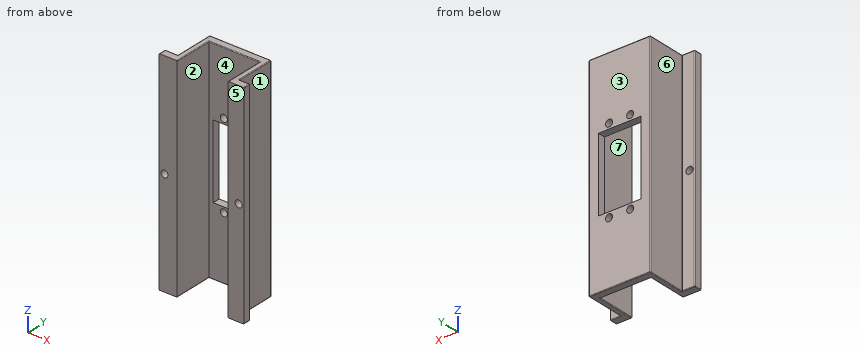
Autodesk Inventor part; units mm, degrees
ref_plane "YZ Plane" through (0, 0, 0) normal (1, 0, 0) x (0, 1, 0)
ref_plane "XZ Plane" through (0, 0, 0) normal (0, 1, 0) x (-1, 0, 0)
ref_plane "XY Plane" through (0, 0, 0) normal (0, 0, 1) x (1, 0, 0)
sketch "Sketch1" plane through (0, 0, 0) normal (0, 1, 0) x (-1, 0, 0)
  line L0 (-40, 0) -> (-40, -100)
  line L1 (0, -100) -> (0, 0)
  line L2 (-35, 0) -> (-35, -100)
  line L3 (-6, -100) -> (-6, 0)
  circle A0 centre (-2.5, -50) radius 1.65
  circle A1 centre (-37.5, -50) radius 1.65
  line L4 (0, 0) -> (-8.5, 0)
  line L5 (-32.5, 0) -> (-40, 0)
  line L6 (-40, -100) -> (-32.5, -100)
  line L7 (-8.5, -100) -> (0, -100)
  line L8 (-8.5, 0) -> (-8.5, -100)
  line L9 (-32.5, -100) -> (-32.5, 0)
  dimension "d4" = 3.3
  dimension "d5" = 3.3
  dimension "d8" = 2.5
  dimension "d9" = 2.5
extrude "Extrusion1" add sketch "Sketch1" along normal blind 3.5
sketch "Sketch2" plane through (0, 3.5, 0) normal (0, 1, 0) x (1, 0, 0)
  line L0 (8.5, 100) -> (0, 100)
  line L1 (8.5, 100) -> (6, 100)
  line L2 (6, 100) -> (6, 0)
  line L3 (6, 0) -> (8.5, 0)
  line L4 (8.5, 0) -> (8.5, 100)
  line L5 (32.5, 100) -> (32.5, 0)
  line L6 (32.5, 100) -> (35, 100)
  line L7 (35, 100) -> (35, 0)
  line L8 (35, 0) -> (32.5, 0)
  line L9 (32.5, 0) -> (32.5, 100)
  point P0 (0, 0)
  point P1 (32.5, 0)
  point P2 (6, 100)
  dimension "d10" = 2.5
  dimension "d11" = 100
  dimension "d12" = 2.5
  dimension "d13" = 100
extrude "Extrusion2" add sketch "Sketch2" along normal blind 15
sketch "Sketch3" plane through (0, 18.5, 0) normal (0, 1, 0) x (1, 0, 0)
  line L0 (6, 100) -> (6, 0)
  line L1 (35, 100) -> (35, 0)
  line L2 (6, 0) -> (35, 0)
  line L3 (35, 0) -> (35, 100)
  line L4 (35, 100) -> (6, 100)
  line L5 (6, 100) -> (6, 0)
  point P0 (0, 0)
  point P1 (35, 0)
  point P2 (6, 100)
extrude "Extrusion3" add sketch "Sketch3" along normal blind 3.5
sketch "Sketch4" plane through (0, 22, 0) normal (0, 1, 0) x (1, 0, 0)
  circle A0 centre (15.5, 70) radius 1.65
  circle A1 centre (25.5, 70) radius 1.65
  circle A2 centre (15.5, 30) radius 1.65
  circle A3 centre (25.5, 30) radius 1.65
  line L0 (30.5, 67.5) -> (10.5, 67.5)
  line L1 (10.5, 67.5) -> (10.5, 32.5)
  line L2 (10.5, 32.5) -> (30.5, 32.5)
  line L3 (30.5, 32.5) -> (30.5, 67.5)
  dimension "d36" = 20
  dimension "d37" = 35
extrude "Extrusion4" cut sketch "Sketch4" against normal blind 3.5
fillet "Fillet1" radius 0.3 24 edges at (6, 12.75, -100) (3, 3.5, -100) (20.5, 22, -100) (8.5, 9.25, -100) (20.5, 18.5, -100) (35, 12.75, -100) (32.5, 9.25, -100) (32.5, 9.25, 0) (35, 12.75, 0) (20.5, 22, 0) (20.5, 18.5, 0) (8.5, 9.25, 0) (6, 12.75, 0) (6, 22, -50) (35, 22, -50) (0, 3.5, -50) (40, 3.5, -50) (37.5, 3.5, 0) (3, 3.5, 0) (0, 1.75, 0) (40, 1.75, 0) (40, 1.75, -100) (37.5, 3.5, -100) (0, 1.75, -100)
fillet "Fillet2" radius 0.3 6 edges at (6.0879, 3.4121, -99.9121) (6.0879, 3.4121, -0.0879) (6, 3.5, -50) (34.9121, 3.4121, -0.0879) (34.9121, 3.4121, -99.9121) (35, 3.5, -50)
properties part number "controllerHousing"
Part model, mm, in its own coordinate system. Face numbers are marked on the shaded views. A direction names the side the tool comes from. Coordinates: 2 decimals unless noted, no trailing zeros. Order: outer loops, then holes, each group sorted by start corner. A loop starts at its lowest first (then second) coordinate and runs counter-clockwise, first axis right, second up. Notation, with made-up numbers: M -12.75,-34.75 L 32.25,-34.75 A28 cw 32.25,-12.75 Z; hole C 87.25,-11 d3. An arc over 180 degrees is marked long. One line per question, with ' | ' between items.
Q1. Slice it at B-B (z = -70). Give the cut face in (x, y).
A:
outline: M 0,0 L 8.5,0 L 8.5,18.5 L 13.85,18.5 L 13.85,22 L 6.3,22 A0.3 ccw 6,21.7 L 6,3.8 A0.3 cw 5.7,3.5 L 0.3,3.5 A0.3 ccw 0,3.2 Z; M 17.15,18.5 L 23.85,18.5 L 23.85,22 L 17.15,22 Z; M 27.15,18.5 L 32.5,18.5 L 32.5,0 L 40,0 L 40,3.2 A0.3 ccw 39.7,3.5 L 35.3,3.5 A0.3 cw 35,3.8 L 35,21.7 A0.3 ccw 34.7,22 L 27.15,22 Z
Q2. Slice it at C-C (x = 25.5). Give the cut face in (y, z), and give its area (3 significant figures).
A:
outline: M 18.5,-99.7 A0.3 ccw 18.8,-100 L 21.7,-100 A0.3 ccw 22,-99.7 L 22,-71.65 L 18.5,-71.65 Z; M 18.5,-68.35 L 22,-68.35 L 22,-67.5 L 18.5,-67.5 Z; M 18.5,-32.5 L 22,-32.5 L 22,-31.65 L 18.5,-31.65 Z; M 18.5,-28.35 L 22,-28.35 L 22,-0.3 A0.3 ccw 21.7,0 L 18.8,0 A0.3 ccw 18.5,-0.3 Z | area: 204 mm^2
Q3. Slice it at D-D (y = 15.75). Give the cut face in (x, z), and give its area (3 significant figures).
A:
outline: M 6,-99.7 A0.3 ccw 6.3,-100 L 8.2,-100 A0.3 ccw 8.5,-99.7 L 8.5,-0.3 A0.3 ccw 8.2,0 L 6.3,0 A0.3 ccw 6,-0.3 Z; M 32.5,-99.7 A0.3 ccw 32.8,-100 L 34.7,-100 A0.3 ccw 35,-99.7 L 35,-0.3 A0.3 ccw 34.7,0 L 32.8,0 A0.3 ccw 32.5,-0.3 Z | area: 500 mm^2
Q4. Slice it at A-A (x = 2.5). Give the cut face in (y, z).
A:
outline: M 0,-100 L 3.2,-100 A0.3 ccw 3.5,-99.7 L 3.5,-51.65 L 0,-51.65 Z; M 0,-48.35 L 3.5,-48.35 L 3.5,-0.3 A0.3 ccw 3.2,0 L 0,0 Z
Q5. 3-axis set-ups, long thin cutter, end or side, ignore diameter. For the marked faces 5, 6 and 7: which of +Z, -Z, +X, -X, +Y, -Y reach the whole face in a straight line?
A:
face 5: +Z, -Z, +X, -X, -Y | face 6: +Z, -Z, -X, +Y | face 7: +Z, -Z, -Y
Q6. Pin check, flat tips, straight feed: P1, Ø1.8, axis at y = 19.5, z = -55, coming from the -X side; P2, Ø4, axis at y = 20, z = -45.5, coming from the +X side; P3, Ø2, axis at x = 15.5, z = -30, coming from the +Y side; P4, Ø6, axis at x = 18.5, z = -67, coming from the -Y side. Stop position of each tip, or through.
A:
P1: stops at x = 6 | P2: stops at x = 35 | P3: passes through | P4: stops at y = 18.5
Q7. Drill centre lines: line 1 (Z direction, x = 15.5, y = 20.3); line 2 (X direction, y = 20.9, z = -70); line 3 (X direction, y = 12, z = -26). Where is each one in solid material? Low to high.
A:
line 1: z = -100 to -71.65, -68.35 to -67.5, -32.5 to -31.65, -28.35 to 0 | line 2: x = 6 to 13.85, 17.15 to 23.85, 27.15 to 35 | line 3: x = 6 to 8.5, 32.5 to 35
Q8. Two-plate mould, pull along X, no slides. Class the marked faces 1, 2, 3 and 4: +X half, -X half, draft (parallel to the pull), parting line (faces both ways), or undercut.
A:
face 1: +X half | face 2: undercut | face 3: draft | face 4: undercut
